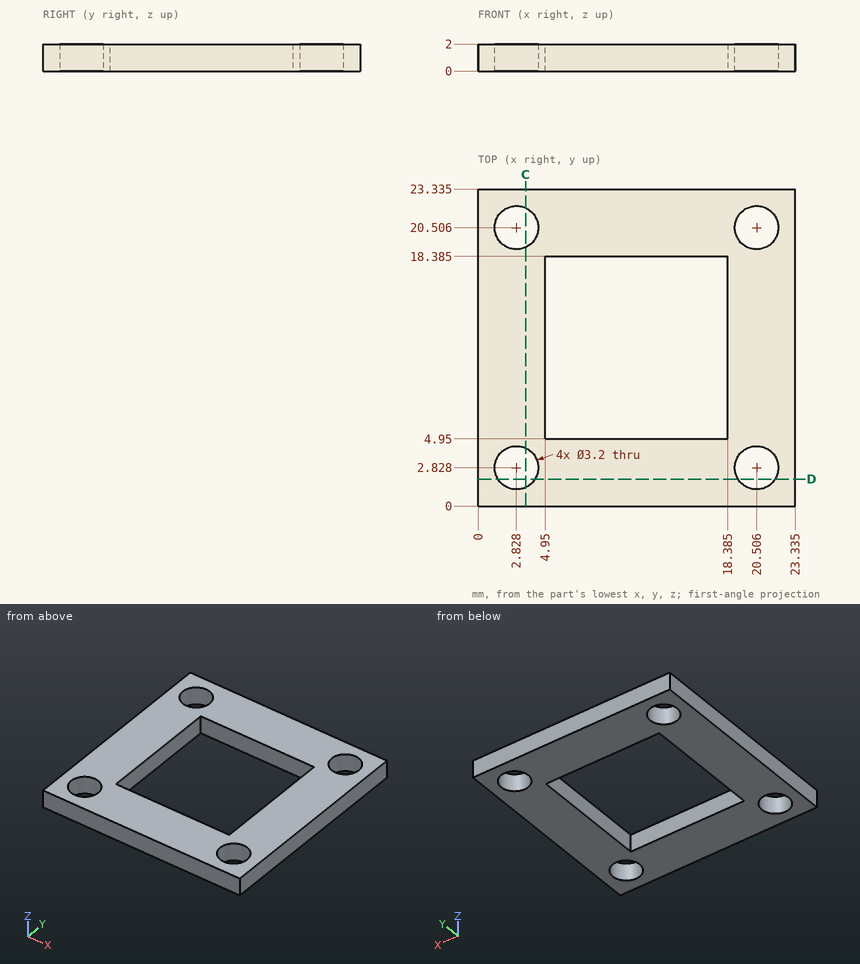
Check sheet for the drawn part. Datum: minimum x, y, z corner. Units: mm. Round coordinates to 2 decimals unless told otherwise and drop trailing zeros. Write each loop counter-clockwise with the first axis right and the second up, starting at its lowest first coordinate (ties: lowest second). Pieces come first, ordered by that corner, then holes. Notation, with made-up numbers: (-39, 86) -> (3, 86) arc R30 ccw to (3, 116) -> close; hole circle Ø7 at (82, -29.75). An arc over 180 degrees is marked (long way). Put each result on its own line as item: value.
(1) Sectioned sample at C-C (x = 3.5). Enter the section's corners in (y, z) (1 decimal).
Values found:
outline: (0, 0) -> (1.4, 0) -> (1.4, 2) -> (0, 2) -> close; (4.3, 0) -> (19.1, 0) -> (19.1, 2) -> (4.3, 2) -> close; (22, 0) -> (23.3, 0) -> (23.3, 2) -> (22, 2) -> close
(2) Go/stop test with a flat-tipped pin: pin 1 Ø1.9 at (x, y) = (20.51, 20.51) entering from +Z. Record where the tip stops, or that it passes through.
Values found:
pin 1: passes through
(3) Sectioned sample at D-D (y = 2). Enter the section's corners in (x, z) (1 decimal).
Values found:
outline: (0, 0) -> (1.5, 0) -> (1.5, 2) -> (0, 2) -> close; (4.2, 0) -> (19.1, 0) -> (19.1, 2) -> (4.2, 2) -> close; (21.9, 0) -> (23.3, 0) -> (23.3, 2) -> (21.9, 2) -> close
(4) Material ranges on line 1 (X direction, y = 4.25, z = 1.05) (1 decimal); line 2 (Y direction, x = 20, z = 1.35) (1 decimal); line 3 (X direction, y = 4, z = 0.55) (1 decimal), recorded low to high.
Values found:
line 1: x = 0 to 2.1, 3.6 to 19.8, 21.2 to 23.3
line 2: y = 0 to 1.3, 4.3 to 19, 22 to 23.3
line 3: x = 0 to 1.7, 3.9 to 19.4, 21.6 to 23.3
